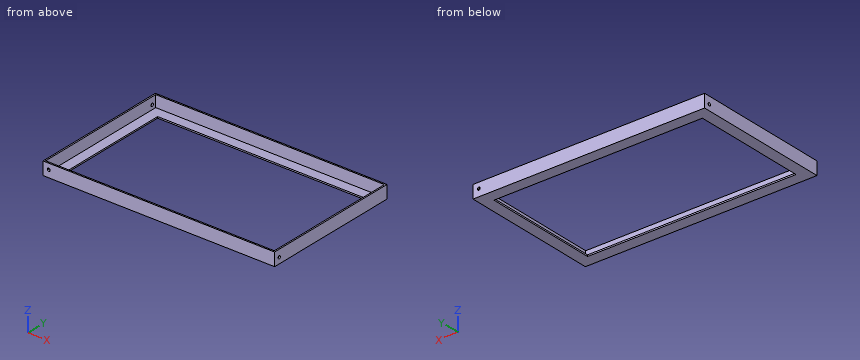
```python
from build123d import *

# Parameters (mm, degrees)
F0_W      = 3.175
F0_H      = 254
F0_H_2    = 22.225
F0_H_3    = 3.175
F0_W_2    = 22.225
F0_W_3    = 457.2
F1_DEPTH  = 25.4
F2_W      = 508
F2_H      = 304.8
F2_W_2    = 501.65
F2_H_2    = 298.45
F2_W_3    = 457.2
F2_H_3    = 254
F3_DEPTH  = 3.175
F5_D      = 6.35
F5_DEPTH  = 12.7
F5_TIP    = 1.9077324654
F7_D      = 6.35
F7_DEPTH  = 12.7
F7_TIP    = 1.9077324654
F9_D      = 6.35
F9_DEPTH  = 12.7
F9_TIP    = 1.9077324654
F11_D     = 6.35
F11_DEPTH = 12.7
F11_TIP   = 1.9077324654


with BuildPart() as f1:
    # F0 (on Top) → F1 (new body)
    with BuildSketch(Plane.XY):
        with Locations((-257.3892009914, 11.9460101733)):
            Rectangle(F0_W, F0_H)
        with Locations((-257.3892009914, -126.1664898267)):
            Rectangle(F0_W, F0_H_2)
        with Locations((-257.3892009914, -138.8664898267)):
            Rectangle(F0_W, F0_H_3)
        with Locations((-244.6892009914, -138.8664898267)):
            Rectangle(F0_W_2, F0_H_3)
        with Locations((-4.9767009914, -138.8664898267)):
            Rectangle(F0_W_3, F0_H_3)
        with Locations((234.7357990086, -138.8664898267)):
            Rectangle(F0_W_2, F0_H_3)
        with Locations((247.4357990086, -138.8664898267)):
            Rectangle(F0_W, F0_H_3)
        with Locations((247.4357990086, -126.1664898267)):
            Rectangle(F0_W, F0_H_2)
        with Locations((247.4357990086, 11.9460101733)):
            Rectangle(F0_W, F0_H)
        with Locations((247.4357990086, 150.0585101733)):
            Rectangle(F0_W, F0_H_2)
        with Locations((247.4357990086, 162.7585101733)):
            Rectangle(F0_W, F0_H_3)
        with Locations((234.7357990086, 162.7585101733)):
            Rectangle(F0_W_2, F0_H_3)
        with Locations((-4.9767009914, 162.7585101733)):
            Rectangle(F0_W_3, F0_H_3)
        with Locations((-244.6892009914, 162.7585101733)):
            Rectangle(F0_W_2, F0_H_3)
        with Locations((-257.3892009914, 162.7585101733)):
            Rectangle(F0_W, F0_H_3)
        with Locations((-257.3892009914, 150.0585101733)):
            Rectangle(F0_W, F0_H_2)
    extrude(amount=F1_DEPTH)

    # F2 (on face) → F3 (join)
    with BuildSketch(Plane(origin=(0, 0, 0), x_dir=(1, 0, 0), z_dir=(0, 0, -1))):
        with Locations((-4.9767009914, -11.9460101733)):
            Rectangle(F2_W, F2_H)
        with Locations((-4.9767009914, -11.9460101733)):
            Rectangle(F2_W_2, F2_H_2, mode=Mode.SUBTRACT)
        with Locations((-4.9767009914, -11.9460101733)):
            Rectangle(F2_W_2, F2_H_2)
        with Locations((-4.9767009914, -11.9460101733)):
            Rectangle(F2_W_3, F2_H_3, mode=Mode.SUBTRACT)
    extrude(amount=F3_DEPTH)

    # F5
    with Locations(Plane.XZ.offset(140.4539898267)):
        with Locations((-246.2767009914, 12.7)):
            Hole(F5_D / 2, depth=F5_DEPTH)
            with Locations((0, 0, -(F5_DEPTH + F5_TIP / 2))):  # 118° drill point
                Cone(0, F5_D / 2, F5_TIP, mode=Mode.SUBTRACT)

    # F7
    with Locations(Plane.YZ.offset(249.0232990086)):
        with Locations((-127.7539898267, 9.525)):
            Hole(F7_D / 2, depth=F7_DEPTH)
            with Locations((0, 0, -(F7_DEPTH + F7_TIP / 2))):  # 118° drill point
                Cone(0, F7_D / 2, F7_TIP, mode=Mode.SUBTRACT)

    # F9
    with Locations(Plane(origin=(0, 164.3460101733, 0), x_dir=(-1, 0, 0), z_dir=(0, 1, 0))):
        with Locations((-236.3232990086, 12.7)):
            Hole(F9_D / 2, depth=F9_DEPTH)
            with Locations((0, 0, -(F9_DEPTH + F9_TIP / 2))):  # 118° drill point
                Cone(0, F9_D / 2, F9_TIP, mode=Mode.SUBTRACT)

    # F11
    with Locations(Plane(origin=(-258.9767009914, 0, 0), x_dir=(0, -1, 0), z_dir=(-1, 0, 0))):
        with Locations((-151.6460101733, 9.525)):
            Hole(F11_D / 2, depth=F11_DEPTH)
            with Locations((0, 0, -(F11_DEPTH + F11_TIP / 2))):  # 118° drill point
                Cone(0, F11_D / 2, F11_TIP, mode=Mode.SUBTRACT)


solid = f1.part
```
For this review, take the finished solid that the model builds, in its own axes (mm). Give positions to 0.01 mm unless a question says otherwise; leave off trailing zeros. Order: outer loops, then holes, each group sorted by start corner. A loop starts at its lowest first (then second) coordinate and runs counter-clockwise, first axis right, second up.
1) Insertion check: pin 1 (5 mm diameter, centred on y = 151.65, z = 9.52, fed in from -X); pin 2 (4 mm diameter, centred on y = -127.75, z = 9.52, fed in from +X). Each pin has a flat end and moves straight along its axis. Give the tip position at first contact, or say it passes through.
2) Take a section at A-A (y = -23). Give the boundary of the cut face in (x, z) (3 decimals), then the cut area to 3 significant figures.
3) Wall thickness on line 1 (Y direction, x = 214.5, z = 10.5); line 2 (X direction, y = 13, z = 11.25); line 3 (X direction, y = -104, z = -1.5): over which ranges is each line inside the solid? List them lowest first.
4) Take a section at B-B (x = 26). Give the boundary of the cut face in (y, z) (3 decimals).
Derived:
1. pin 1: stops at x = 245.85
1. pin 2: stops at x = -255.8
2. outline: (-258.977, -3.175) - (-233.577, -3.175) - (-233.577, 0) - (-255.802, 0) - (-255.802, 25.4) - (-258.977, 25.4) - close; (223.623, -3.175) - (249.023, -3.175) - (249.023, 25.4) - (245.848, 25.4) - (245.848, 0) - (223.623, 0) - close
2. area: 323 mm2
3. line 1: y = -140.45 to -137.28, 161.17 to 164.35
3. line 2: x = -258.98 to -255.8, 245.85 to 249.02
3. line 3: x = -258.98 to -233.58, 223.62 to 249.02
4. outline: (-140.454, -3.175) - (-115.054, -3.175) - (-115.054, 0) - (-137.279, 0) - (-137.279, 25.4) - (-140.454, 25.4) - close; (138.946, -3.175) - (164.346, -3.175) - (164.346, 25.4) - (161.171, 25.4) - (161.171, 0) - (138.946, 0) - close
